Can you work these out from the model? Positions are in its coordinate system, mm. Face numbers are marked on the shaded views. A direction names the side the tool comes from. Coordinates: 2 decimals unless noted, no trailing zeros. Write each loop counter-clockwise with the first axis right and the second up, starting at its lowest first coordinate (ties: lowest second). Pieces come first, ordered by that corner, then holes. Notation, with made-up numbers: (45, -9.5) - (100, -9.5) arc R12 ccw to (100, 13.5) - close; hole circle Ø5 at (-29.5, 82.25). An arc over 180 degrees is marked (long way). One line per question, with ' | ' between items. Start each with the question number.
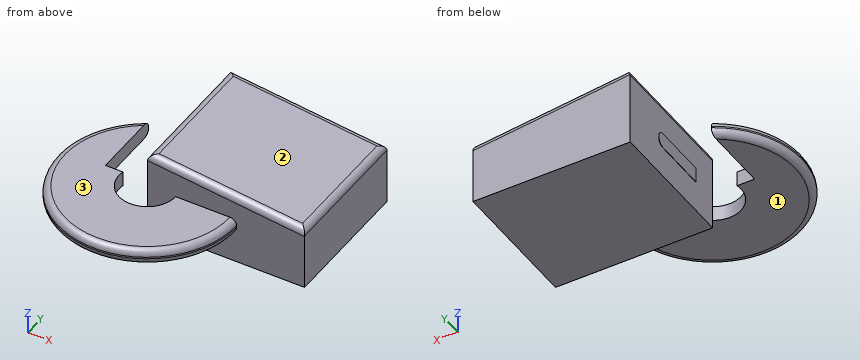
from build123d import *

# Parameters (mm, degrees)
F1_DEPTH = 102.6981025934
F4_R     = 5.08
F5_W     = 33.7471216917
F5_H     = 65.5695050955
F6_DEPTH = 25.4


with BuildPart() as f1:
    # F0 (on Front) → F1 (new body)
    with BuildSketch(Plane.XZ):
        Polygon((62.229424715, -34.6546843648), (62.229424715, 12.4018825591), (-55.8673739433, 26.1995047331), (-55.8673739433, -34.6546843648), align=None)
    extrude(amount=F1_DEPTH)

    # F2 (on face) → F3 (revolve)
    with BuildSketch(Plane.XZ.offset(102.6981025934)):
        Polygon((-34.6154049039, -11.3538783044), (11.5415975451, -11.3538783044), (11.0295861959, 0), (-34.6154049039, 0), align=None)
    revolve(axis=Axis((-55.8673739433, -102.6981025934, -4.2275898159), (0, 0, 1)))

    # F4
    f4_edges = [f1.edges().sort_by_distance(p)[0] for p in [
        (62.229425, -51.349051, 12.401883),
        (-55.867374, -51.349051, 26.199505),
        (3.181025, 0, 19.300694),
        (3.181025, -102.698103, 19.300694),
        (-103.532715, -150.363443, -11.353878),
        (-103.170668, -150.001397, 0),
    ]]
    fillet(f4_edges, radius=F4_R)

    # F5 (on Top) → F6 (cut)
    with BuildSketch(Plane.XY):
        with Locations((-72.9322209954, -65.7769069076)):
            Rectangle(F5_W, F5_H)
    extrude(amount=-F6_DEPTH, mode=Mode.SUBTRACT)


solid = f1.part
(1) If we section it at A-A on y = -32: List the corners of the cut face in (x, z) for me, plus the area to 3 significant figures.
(2) Which directions (+Z, -Z, +X, -X, +Y, -Y) give clear straight access to the entire face, cutting with the end or side of a thin tool? Please do the marked faces 1, 2 and 3.
(3) I'm going to push flat-ended pins straight in: pin 1 (3 mm diameter, centred on y = -132.5, z = -6.5, fed in from +X); pin 2 (16.5 mm diameter, centred on y = -67.5, z = -3, fed in from -X); pin 3 (12.5 mm diameter, centred on y = -66.5, z = -4, fed in from -X). Where does each tip first touch, or does it pass through?
(4) If I drill on probe 1 along Z at (x, y) = (-8.5, -116); probe 2 along Y at (x, z) = (55.5, 3.5); probe 3 along X at (y, z) = (-88.5, -8), over which ranges is the centre line in solid material (lowest first)?
(5) If we section it at C-C on z = -21: List the corners of the cut face in (x, y) for me, plus the area to 3 significant figures.
(6) If we section it at B-B on z = -9: List the corners of the cut face in (x, y) for me.
Values:
1) outline: (-55.87, -34.65) - (62.23, -34.65) - (62.23, 7.88) arc R5.08 ccw to (57.74, 12.93) - (-50.2, 25.54) arc R5.08 ccw to (-55.87, 20.49) - close | area: 6,360 mm2
2) face 1: -Z, -X, -Y | face 2: +Z, +X, +Y, -Y | face 3: +Z, -X, -Y
3) pin 1: x = 5.05 | pin 2: x = -117.25 | pin 3: x = -115.9
4) probe 1: -11.35 to 0 | probe 2: -102.7 to 0 | probe 3: -121.22 to -89.81, -55.87 to 62.23
5) outline: (-55.87, -102.7) - (62.23, -102.7) - (62.23, 0) - (-55.87, 0) - close | area: 12,100 mm2
6) outline: (-89.81, -98.56) - (-89.81, -45.65) arc R66.38 ccw (long way) to (10.51, -102.7) - (62.23, -102.7) - (62.23, 0) - (-55.87, 0) - (-55.87, -36.32) arc R66.38 ccw to (-56.06, -36.32) - (-56.06, -81.45) arc R21.25 cw to (-55.87, -81.45) - (-55.87, -102.7) - (-34.62, -102.7) arc R21.25 cw (long way) to (-76.71, -98.56) - close
